```python
from build123d import *

# Parameters (mm, degrees)
F1_R     = 3.5
F1_R_2   = 3
F1_R_3   = 1.45
F2_DEPTH = 1


with BuildPart() as f2:
    # F1 (on Top) → F2 (new body)
    with BuildSketch(Plane.XY):
        with BuildLine():
            add(Edge.make_bspline(
                [(4.2, 8), (4.2, 4.3558003341), (4.3243523603, 4.2), (9.5, 4.2)],
                knots=[0, 0, 0, 0, 6.5215028943, 6.5215028943, 6.5215028943, 6.5215028943], degree=3))
            ThreePointArc((4.2, 8), (0, 3.8), (-4.2, 8))
            add(Edge.make_bspline(
                [(-4.2, 8), (-4.2, 4.3558003341), (-4.3243523603, 4.2), (-9.5, 4.2)],
                knots=[0, 0, 0, 0, 6.5215028943, 6.5215028943, 6.5215028943, 6.5215028943], degree=3))
            ThreePointArc((-9.5, 4.2), (-6.530151519, 2.969848481), (-5.3, 0))
            ThreePointArc((-5.3, 0), (-6.530151519, -2.969848481), (-9.5, -4.2))
            add(Edge.make_bspline(
                [(-4.2, -8), (-4.2, -4.3558003341), (-4.3243523603, -4.2), (-9.5, -4.2)],
                knots=[0, 0, 0, 0, 6.5215028943, 6.5215028943, 6.5215028943, 6.5215028943], degree=3))
            ThreePointArc((-4.2, -8), (0, -3.8), (4.2, -8))
            add(Edge.make_bspline(
                [(9.5, -4.2), (4.3243523603, -4.2), (4.2, -4.3558003341), (4.2, -8)],
                knots=[0, 0, 0, 0, 6.5215028943, 6.5215028943, 6.5215028943, 6.5215028943], degree=3))
            ThreePointArc((9.5, -4.2), (5.3, 0), (9.5, 4.2))
        make_face()
        Circle(F1_R, mode=Mode.SUBTRACT)
        with BuildLine():
            ThreePointArc((-5.3, 0), (-6.530151519, 2.969848481), (-9.5, 4.2))
            ThreePointArc((-9.5, 4.2), (-13.7, 0), (-9.5, -4.2))
            ThreePointArc((-9.5, -4.2), (-6.530151519, -2.969848481), (-5.3, 0))
        make_face()
        with Locations((-9.5, 0)):
            Circle(F1_R_2, mode=Mode.SUBTRACT)
        with BuildLine():
            ThreePointArc((-4.2, -8), (0, -12.2), (4.2, -8))
            ThreePointArc((4.2, -8), (0, -3.8), (-4.2, -8))
        make_face()
        with Locations((0, -8)):
            Circle(F1_R_2, mode=Mode.SUBTRACT)
        with BuildLine():
            ThreePointArc((13.7, 0), (12.469848481, 2.969848481), (9.5, 4.2))
            ThreePointArc((9.5, 4.2), (5.3, 0), (9.5, -4.2))
            ThreePointArc((9.5, -4.2), (12.469848481, -2.969848481), (13.7, 0))
        make_face()
        with Locations((9.5, 0)):
            Circle(F1_R_2, mode=Mode.SUBTRACT)
        with BuildLine():
            ThreePointArc((-4.2, 8), (0, 3.8), (4.2, 8))
            ThreePointArc((4.2, 8), (0, 12.2), (-4.2, 8))
        make_face()
        with Locations((0, 8)):
            Circle(F1_R_2, mode=Mode.SUBTRACT)
        with Locations((0, 8)):
            Circle(F1_R_2)
        with Locations((0, 8)):
            Circle(F1_R_3, mode=Mode.SUBTRACT)
        with Locations((-9.5, 0)):
            Circle(F1_R_2)
        with Locations((-9.5, 0)):
            Circle(F1_R_3, mode=Mode.SUBTRACT)
        with Locations((0, -8)):
            Circle(F1_R_2)
        with Locations((0, -8)):
            Circle(F1_R_3, mode=Mode.SUBTRACT)
        with Locations((9.5, 0)):
            Circle(F1_R_2)
        with Locations((9.5, 0)):
            Circle(F1_R_3, mode=Mode.SUBTRACT)
    extrude(amount=F2_DEPTH)


solid = f2.part
```
Work out the finished part from the listing and answer in its coordinate system (mm). Give positions to 0.01 mm unless a question says otherwise; leave off trailing zeros. Loops run counter-clockwise (first coordinate to the right, second up) from the corner with the lowest first, then second, coordinate; pieces in that order, holes last. Notation, with made-up numbers: (79, 35) -> (132, 35) arc R28 cw to (132, 56) -> close; hole circle Ø10 at (24.25, -36). An arc over 180 degrees is marked (long way). Write item = value, one per line. Start each with the question number.
(1) Find section C-C on y = -10.25. Give the vertices of the cut face in (x, z), and give its area (3 significant figures).
(2) The mould has two halves that part along Y. Classify faces 1 (the flat face through (-3, -3, 1)), 2 (the cylindrical face through (-13.7, 0.1, 0.5)), 3 (the cylindrical face through (-0.314, 6.584, 0.493)): +Y half, -Y half, draft (parallel to the pull), parting line (faces both ways), or undercut.
(3) Find the intervals of material crossed by probe 1 along Y at (x, z) = (0, 0.4); probe 2 along X at (y, z) = (0.25, 0.7); probe 3 along Y at (x, z) = (9.5, 0.5), in increasing order. Write a range as from..to.
(4) Find section A-A on x = 0. Give the vertices of the cut face in (y, z), and give its area (3 significant figures).
(5) Find section D-D on x = 11.25. Give the vertices of the cut face in (y, z), and give its area (3 significant figures).
(6) Find section B-B on z = 0.4. Give the number of separate pieces and of enclosed holes in the cut face, and give its area (3 significant figures).
(7) Given pin 1 Ø2.5 at (x, y) = (0, 8) entering from +Z, flat-ended and moving along its own axis, determine where the tip first touches the part or whether it passes through.
From the geometry:
q1.outline = (-3.55, 0) -> (3.55, 0) -> (3.55, 1) -> (-3.55, 1) -> close
q1.area = 7.09 mm^2
q2.face_1 = draft
q2.face_2 = parting line
q2.face_3 = undercut
q3.probe_1 = -12.2..-9.45, -6.55..-3.5, 3.5..6.55, 9.45..12.2
q3.probe_2 = -13.69..-10.93, -8.07..-3.49, 3.49..8.07, 10.93..13.69
q3.probe_3 = -4.2..-1.45, 1.45..4.2
q4.outline = (-12.2, 0) -> (-9.45, 0) -> (-9.45, 1) -> (-12.2, 1) -> close; (-6.55, 0) -> (-3.5, 0) -> (-3.5, 1) -> (-6.55, 1) -> close; (3.5, 0) -> (6.55, 0) -> (6.55, 1) -> (3.5, 1) -> close; (9.45, 0) -> (12.2, 0) -> (12.2, 1) -> (9.45, 1) -> close
q4.area = 11.6 mm^2
q5.outline = (-3.82, 0) -> (3.82, 0) -> (3.82, 1) -> (-3.82, 1) -> close
q5.area = 7.64 mm^2
q6.separate_pieces = 1
q6.enclosed_holes = 5
q6.area = 274 mm^2
q7.pin_1 = through
